```python
from build123d import *

# Parameters (mm, degrees)
SKETCH2_R               = 0.875
BOLT_HOLE_DEPTH         = 3
BOLT_HOLE_PATTERN_COUNT = 6


with BuildPart() as part:
    # Nozzle base structure → Revolve1 (revolve)
    with BuildSketch(Plane(origin=(0, 0, 0), x_dir=(0, 0, -1), z_dir=(1, 0, 0)), mode=Mode.PRIVATE) as revolve1_sk:
        Polygon((0, 4.5), (72.97, 24.553), (72.97, 27.445755495), (72.175037331, 27.445755495), (0.935060955, 7.868185997), (-8.714285714, 18), (-25, 18), (-25, 23), (-28, 23), (-28, 18), (-28, 10), (-25, 10), (-25, 15), (-10, 15), align=None)
    revolve(revolve1_sk.sketch.rotate(Axis((0, 0, 0), (0, 0, -1)), 90), axis=Axis((0, 0, 0), (0, 0, -1)))

    # Throat
    # a fillet whose section is not a circle: 10 mm, written as the material it takes off along each edge
    with BuildSketch(Plane(origin=(0, 0, 0), x_dir=(1, 0, 0), z_dir=(0, 1, 0))) as throat_piece_1:
        with BuildLine():
            Bezier((6.08476834, 5.766745413), (4.5, 0), (8.830734933, -4.12450946), weights=[1, 1.857142857, 1])
            Line((8.830734933, -4.12450946), (4.5, 0))
            Line((4.5, 0), (6.08476834, 5.766745413))
        make_face()
    revolve(axis=Axis((0, 0, 0), (0, 0, -1)), mode=Mode.SUBTRACT)

    # Sketch2 → Bolt hole (cut)
    with BuildSketch(Plane(origin=(0, 0, 25), x_dir=(-1, 0, 0), z_dir=(0, 0, -1))):
        with Locations((0, 20.5)):
            Circle(SKETCH2_R)
    bolt_hole = extrude(amount=-BOLT_HOLE_DEPTH, mode=Mode.SUBTRACT)

    # Bolt hole pattern: Bolt hole ×6 about axis
    bolt_hole_pattern_axis = Axis((0, 0, 0), (0, 0, 1))
    for i in range(1, BOLT_HOLE_PATTERN_COUNT):
        add(bolt_hole.rotate(bolt_hole_pattern_axis, i * 360 / BOLT_HOLE_PATTERN_COUNT), mode=Mode.SUBTRACT)


solid = part.part
```
Geometry check sheet. Reference: the model listing, model coordinates, mm. A direction names the side the tool comes from. Round coordinates to 2 decimals unless told otherwise and drop trailing zeros. Write each loop counter-clockwise with the first axis right and the second up, starting at its lowest first coordinate (ties: lowest second). Pieces come first, ordered by that corner, then holes. Notation, with made-up numbers: (-5.5, 49) -> (8.5, 49) arc R16 ccw to (8.5, 70) -> close; hole circle Ø7 at (51.5, 11). An arc over 180 degrees is marked (long way). Put each result on its own line as item: value.
1) Thickness scan on probe 1 along Y at (x, z) = (0, 26.3) (3 decimals); probe 2 along Y at (x, z) = (-3, -48); probe 3 along Y at (x, z) = (14, -67). Record the ranges inside material, lowest first. Write a range as from..to.
Recorded:
probe 1: y = -23..-21.375, -19.625..-10, 10..19.625, 21.375..23
probe 2: y = -20.58..-17.43, 17.43..20.58
probe 3: y = -21.94..-18.14, 18.14..21.94
2) Release check for a two-part mould opening along Z. For faces 1 (the face through (-5.95, 26.793, -72.567)), 2 (the face through (-13.267, -12.165, 16.971)), 3 (the face through (20.5, 14.1, -72.97)), 4 (the face through (8.71, -2.74, 4.41)) record: pulls with the +Z half, pulls with the -Z half, needs draft (parallel to the pull), parting line crosses it, or undercut.
Recorded:
face 1: needs draft
face 2: undercut
face 3: pulls with the -Z half
face 4: undercut
3) Cross-section at A-A, the plane z = 21. Enter the section's corners in (x, y), plus the area to 3 significant figures.
Recorded:
outline: circle Ø36 at (0, 0); hole circle Ø30 at (0, 0)
area: 311 mm2
4) Depth check by flat-ended pin: P1, Ø6, axis at x = -9, z = -26, coming from the +Y side; P2, Ø3, axis at y = -9, z = 2.5, coming from the -X side; P3, Ø10, axis at x = -5, z = -49, coming from the +Y side; P4, Ø12, axis at y = -22, z = -20.5, coming from the +X side. Enter the tip coordinate at first touch or a pass-through.
Recorded:
P1: stops at y = 13.75
P2: stops at x = -9.84
P3: stops at y = 22.13
P4: passes through
5) Access from +Z, -Z, +X, -X, +Y, -Y to the whole of each face (thin tool, end or side, straight path). Record for faces 5 (the face through (-10, 0, 26)), 6 (the face through (8.25, -12.94, -28.14)), 7 (the face through (10, 5, 28)).
Recorded:
face 5: +Z
face 6: none
face 7: +Z, +X, -X, +Y, -Y
6) Cross-section at C-C, the plane z = -39. Enter the section's corners in (x, y).
Recorded:
outline: circle Ø36.66 at (0, 0); hole circle Ø30.44 at (0, 0)
7) Cross-section at B-B, the plane y = -13. Give the number of separate pieces and of enclosed holes in the cut face, plus the area to 3 significant figures.
Recorded:
separate pieces: 2
enclosed holes: 1
area: 865 mm2
